```python
from build123d import *

# Parameters (mm, degrees)
SKETCH1_R                                           = 28
BOSS_EXTRUDE1_DEPTH                                 = 22
SKETCH2_R                                           = 10
BOSS_EXTRUDE2_DEPTH                                 = 22
SKETCH3_R                                           = 20
CUT_EXTRUDE1_DEPTH                                  = 16
CHAMFER1_SIZE                                       = 4
SKETCH4_R                                           = 4
CUT_EXTRUDE2_DEPTH                                  = 20
CBORE_FOR_M3_HEX_SOCKET_HEAD_CAP_SCREW1_D           = 3.4
CBORE_FOR_M3_HEX_SOCKET_HEAD_CAP_SCREW1_CBORE_D     = 6.5
CBORE_FOR_M3_HEX_SOCKET_HEAD_CAP_SCREW1_CBORE_DEPTH = 3.4
SKETCH7_R                                           = 26.5
SKETCH7_R_2                                         = 24.5
CUT_EXTRUDE3_DEPTH                                  = 4
M2_TAPPED_HOLE1_AT_2_COUNT                          = 2
M2_TAPPED_HOLE1_AT_2_PITCH                          = 11.388037985
M2_TAPPED_HOLE1_AT_3_COUNT                          = 2
M2_TAPPED_HOLE1_AT_3_PITCH                          = 22
M2_TAPPED_HOLE1_AT_4_COUNT                          = 2
M2_TAPPED_HOLE1_AT_4_PITCH                          = 31.112698372
M2_TAPPED_HOLE1_AT_5_COUNT                          = 2
M2_TAPPED_HOLE1_AT_5_PITCH                          = 38.105117767
M2_TAPPED_HOLE1_AT_6_COUNT                          = 2
M2_TAPPED_HOLE1_AT_6_PITCH                          = 42.500736357
M2_TAPPED_HOLE1_AT_7_COUNT                          = 2
M2_TAPPED_HOLE1_AT_7_PITCH                          = 44
M2_TAPPED_HOLE1_AT_8_COUNT                          = 2
M2_TAPPED_HOLE1_AT_8_PITCH                          = 42.500736357
M2_TAPPED_HOLE1_AT_9_COUNT                          = 2
M2_TAPPED_HOLE1_AT_9_PITCH                          = 38.105117767
M2_TAPPED_HOLE1_AT_10_COUNT                         = 2
M2_TAPPED_HOLE1_AT_10_PITCH                         = 31.112698372
M2_TAPPED_HOLE1_AT_11_COUNT                         = 2
M2_TAPPED_HOLE1_AT_11_PITCH                         = 22
M2_TAPPED_HOLE1_AT_12_COUNT                         = 2
M2_TAPPED_HOLE1_AT_12_PITCH                         = 11.388037985
SKETCH10_R                                          = 28
SKETCH10_R_2                                        = 24
CUT_EXTRUDE5_DEPTH                                  = 6
CUT_EXTRUDE5_DEPTH_BACK                             = 6
CHAMFER2_SIZE                                       = 1
M4_TAPPED_HOLE1_REACH                               = 60.172
M4_TAPPED_HOLE1_BORE_R                              = 1.65
CIRPATTERN1_COUNT                                   = 2
CIRPATTERN1_ANGLE                                   = 90


with BuildPart() as part:
    # Sketch1 → Boss-Extrude1 (new body)
    with BuildSketch(Plane.XY):
        Circle(SKETCH1_R)
    extrude(amount=BOSS_EXTRUDE1_DEPTH)

    # Sketch2 → Boss-Extrude2 (add)
    with BuildSketch(Plane.XY.offset(22)):
        Circle(SKETCH2_R)
    extrude(amount=BOSS_EXTRUDE2_DEPTH)

    # Sketch3 → Cut-Extrude1 (cut)
    with BuildSketch(Plane(origin=(0, 0, 0), x_dir=(-1, 0, 0), z_dir=(0, 0, -1))):
        Circle(SKETCH3_R)
    extrude(amount=-CUT_EXTRUDE1_DEPTH, mode=Mode.SUBTRACT)

    # Chamfer1
    chamfer1_edges = [part.edges().sort_by_distance(p)[0] for p in [
        (20, 0, 16),
    ]]
    chamfer(chamfer1_edges, length=CHAMFER1_SIZE)

    # Sketch4 → Cut-Extrude2 (cut)
    with BuildSketch(Plane.XY.offset(44)):
        Circle(SKETCH4_R)
    extrude(amount=-CUT_EXTRUDE2_DEPTH, mode=Mode.SUBTRACT)

    # CBORE for M3 Hex Socket Head Cap Screw1 (through all)
    with Locations(Plane(origin=(0, 0, 16), x_dir=(-1, 0, 0), z_dir=(0, 0, -1))):
        with Locations((0, 0)):
            CounterBoreHole(CBORE_FOR_M3_HEX_SOCKET_HEAD_CAP_SCREW1_D / 2, CBORE_FOR_M3_HEX_SOCKET_HEAD_CAP_SCREW1_CBORE_D / 2, CBORE_FOR_M3_HEX_SOCKET_HEAD_CAP_SCREW1_CBORE_DEPTH)

    # Sketch7 → Cut-Extrude3 (cut)
    with BuildSketch(Plane(origin=(0, 0, 0), x_dir=(-1, 0, 0), z_dir=(0, 0, -1))):
        Circle(SKETCH7_R)
        Circle(SKETCH7_R_2, mode=Mode.SUBTRACT)
    cut_extrude3 = extrude(amount=-CUT_EXTRUDE3_DEPTH, mode=Mode.SUBTRACT)

    # Mirror1: Cut-Extrude3 across plane
    add(cut_extrude3.mirror(Plane(origin=(0, 0, 11), x_dir=(1, 0, 0), z_dir=(0, 0, -1))), mode=Mode.SUBTRACT)

    # Sketch9 → M2 Tapped Hole1 (revolve, cut)
    with BuildSketch(Plane(origin=(0, 22, 0), x_dir=(0, 1, 0), z_dir=(1, 0, 0))):
        Polygon((0, 0), (0, 8.480688495), (0.8, 8), (0.8, 0), align=None)
    m2_tapped_hole1 = revolve(axis=Axis((0, 22, -6.35), (0, 0, 1)), mode=Mode.SUBTRACT)

    # M2 Tapped Hole1 at 2: M2 Tapped Hole1 ×2
    with Locations(*[Vector(-0.9659258262891051, -0.2588190451023836, 0) * (i * M2_TAPPED_HOLE1_AT_2_PITCH) for i in range(1, M2_TAPPED_HOLE1_AT_2_COUNT)]):
        add(m2_tapped_hole1, mode=Mode.SUBTRACT)

    # M2 Tapped Hole1 at 3: M2 Tapped Hole1 ×2
    with Locations(*[Vector(-0.8660254037845097, -0.4999999999998771, 0) * (i * M2_TAPPED_HOLE1_AT_3_PITCH) for i in range(1, M2_TAPPED_HOLE1_AT_3_COUNT)]):
        add(m2_tapped_hole1, mode=Mode.SUBTRACT)

    # M2 Tapped Hole1 at 4: M2 Tapped Hole1 ×2
    with Locations(*[Vector(-0.7071067811866479, -0.7071067811864472, 0) * (i * M2_TAPPED_HOLE1_AT_4_PITCH) for i in range(1, M2_TAPPED_HOLE1_AT_4_COUNT)]):
        add(m2_tapped_hole1, mode=Mode.SUBTRACT)

    # M2 Tapped Hole1 at 5: M2 Tapped Hole1 ×2
    with Locations(*[Vector(-0.500000000000123, -0.8660254037843677, 0) * (i * M2_TAPPED_HOLE1_AT_5_PITCH) for i in range(1, M2_TAPPED_HOLE1_AT_5_COUNT)]):
        add(m2_tapped_hole1, mode=Mode.SUBTRACT)

    # M2 Tapped Hole1 at 6: M2 Tapped Hole1 ×2
    with Locations(*[Vector(-0.2588190451026581, -0.9659258262890316, 0) * (i * M2_TAPPED_HOLE1_AT_6_PITCH) for i in range(1, M2_TAPPED_HOLE1_AT_6_COUNT)]):
        add(m2_tapped_hole1, mode=Mode.SUBTRACT)

    # M2 Tapped Hole1 at 7: M2 Tapped Hole1 ×2
    with Locations(*[(0, -i * M2_TAPPED_HOLE1_AT_7_PITCH, 0) for i in range(1, M2_TAPPED_HOLE1_AT_7_COUNT)]):
        add(m2_tapped_hole1, mode=Mode.SUBTRACT)

    # M2 Tapped Hole1 at 8: M2 Tapped Hole1 ×2
    with Locations(*[Vector(0.25881904510238346, -0.9659258262891051, 0) * (i * M2_TAPPED_HOLE1_AT_8_PITCH) for i in range(1, M2_TAPPED_HOLE1_AT_8_COUNT)]):
        add(m2_tapped_hole1, mode=Mode.SUBTRACT)

    # M2 Tapped Hole1 at 9: M2 Tapped Hole1 ×2
    with Locations(*[Vector(0.4999999999998768, -0.8660254037845098, 0) * (i * M2_TAPPED_HOLE1_AT_9_PITCH) for i in range(1, M2_TAPPED_HOLE1_AT_9_COUNT)]):
        add(m2_tapped_hole1, mode=Mode.SUBTRACT)

    # M2 Tapped Hole1 at 10: M2 Tapped Hole1 ×2
    with Locations(*[Vector(0.7071067811864471, -0.7071067811866479, 0) * (i * M2_TAPPED_HOLE1_AT_10_PITCH) for i in range(1, M2_TAPPED_HOLE1_AT_10_COUNT)]):
        add(m2_tapped_hole1, mode=Mode.SUBTRACT)

    # M2 Tapped Hole1 at 11: M2 Tapped Hole1 ×2
    with Locations(*[Vector(0.8660254037843675, -0.5000000000001233, 0) * (i * M2_TAPPED_HOLE1_AT_11_PITCH) for i in range(1, M2_TAPPED_HOLE1_AT_11_COUNT)]):
        add(m2_tapped_hole1, mode=Mode.SUBTRACT)

    # M2 Tapped Hole1 at 12: M2 Tapped Hole1 ×2
    with Locations(*[Vector(0.9659258262890317, -0.2588190451026578, 0) * (i * M2_TAPPED_HOLE1_AT_12_PITCH) for i in range(1, M2_TAPPED_HOLE1_AT_12_COUNT)]):
        add(m2_tapped_hole1, mode=Mode.SUBTRACT)

    # Sketch10 → Cut-Extrude5 (cut, two sides)
    with BuildSketch(Plane(origin=(0, 0, 11), x_dir=(-1, 0, 0), z_dir=(0, 0, -1))) as cut_extrude5_sk:
        Circle(SKETCH10_R)
        Circle(SKETCH10_R_2, mode=Mode.SUBTRACT)
    extrude(amount=CUT_EXTRUDE5_DEPTH, mode=Mode.SUBTRACT)
    extrude(cut_extrude5_sk.sketch, amount=-CUT_EXTRUDE5_DEPTH_BACK, mode=Mode.SUBTRACT)

    # Mirror2: M2 Tapped Hole1 across plane
    add(m2_tapped_hole1.mirror(Plane(origin=(0, 0, 11), x_dir=(1, 0, 0), z_dir=(0, 0, -1))), mode=Mode.SUBTRACT)

    # Mirror2 copy 1 sketch → Mirror2 copy 1 (revolve, cut)
    with BuildSketch(Plane(origin=(-11, 19.052558883, 22), x_dir=(0, 1, 0), z_dir=(1, 0, 0))):
        Polygon((0, 0), (0, -8.480688495), (0.8, -8), (0.8, 0), align=None)
    revolve(axis=Axis((-11, 19.052558883, 28.35), (0, 0, 1)), mode=Mode.SUBTRACT)

    # Mirror2 copy 2 sketch → Mirror2 copy 2 (revolve, cut)
    with BuildSketch(Plane(origin=(-19.052558883, 11, 22), x_dir=(0, 1, 0), z_dir=(1, 0, 0))):
        Polygon((0, 0), (0, -8.480688495), (0.8, -8), (0.8, 0), align=None)
    revolve(axis=Axis((-19.052558883, 11, 28.35), (0, 0, 1)), mode=Mode.SUBTRACT)

    # Mirror2 copy 3 sketch → Mirror2 copy 3 (revolve, cut)
    with BuildSketch(Plane(origin=(-22, 0, 22), x_dir=(0, 1, 0), z_dir=(1, 0, 0))):
        Polygon((0, 0), (0, -8.480688495), (0.8, -8), (0.8, 0), align=None)
    revolve(axis=Axis((-22, 0, 28.35), (0, 0, 1)), mode=Mode.SUBTRACT)

    # Mirror2 copy 4 sketch → Mirror2 copy 4 (revolve, cut)
    with BuildSketch(Plane(origin=(-19.052558883, -11, 22), x_dir=(0, 1, 0), z_dir=(1, 0, 0))):
        Polygon((0, 0), (0, -8.480688495), (0.8, -8), (0.8, 0), align=None)
    revolve(axis=Axis((-19.052558883, -11, 28.35), (0, 0, 1)), mode=Mode.SUBTRACT)

    # Mirror2 copy 5 sketch → Mirror2 copy 5 (revolve, cut)
    with BuildSketch(Plane(origin=(-11, -19.052558883, 22), x_dir=(0, 1, 0), z_dir=(1, 0, 0))):
        Polygon((0, 0), (0, -8.480688495), (0.8, -8), (0.8, 0), align=None)
    revolve(axis=Axis((-11, -19.052558883, 28.35), (0, 0, 1)), mode=Mode.SUBTRACT)

    # Mirror2 copy 6 sketch → Mirror2 copy 6 (revolve, cut)
    with BuildSketch(Plane(origin=(0, -22, 22), x_dir=(0, 1, 0), z_dir=(1, 0, 0))):
        Polygon((0, 0), (0, -8.480688495), (0.8, -8), (0.8, 0), align=None)
    revolve(axis=Axis((0, -22, 28.35), (0, 0, 1)), mode=Mode.SUBTRACT)

    # Mirror2 copy 7 sketch → Mirror2 copy 7 (revolve, cut)
    with BuildSketch(Plane(origin=(11, -19.052558883, 22), x_dir=(0, 1, 0), z_dir=(1, 0, 0))):
        Polygon((0, 0), (0, -8.480688495), (0.8, -8), (0.8, 0), align=None)
    revolve(axis=Axis((11, -19.052558883, 28.35), (0, 0, 1)), mode=Mode.SUBTRACT)

    # Mirror2 copy 8 sketch → Mirror2 copy 8 (revolve, cut)
    with BuildSketch(Plane(origin=(19.052558883, -11, 22), x_dir=(0, 1, 0), z_dir=(1, 0, 0))):
        Polygon((0, 0), (0, -8.480688495), (0.8, -8), (0.8, 0), align=None)
    revolve(axis=Axis((19.052558883, -11, 28.35), (0, 0, 1)), mode=Mode.SUBTRACT)

    # Mirror2 copy 9 sketch → Mirror2 copy 9 (revolve, cut)
    with BuildSketch(Plane(origin=(22, 0, 22), x_dir=(0, 1, 0), z_dir=(1, 0, 0))):
        Polygon((0, 0), (0, -8.480688495), (0.8, -8), (0.8, 0), align=None)
    revolve(axis=Axis((22, 0, 28.35), (0, 0, 1)), mode=Mode.SUBTRACT)

    # Mirror2 copy 10 sketch → Mirror2 copy 10 (revolve, cut)
    with BuildSketch(Plane(origin=(19.052558883, 11, 22), x_dir=(0, 1, 0), z_dir=(1, 0, 0))):
        Polygon((0, 0), (0, -8.480688495), (0.8, -8), (0.8, 0), align=None)
    revolve(axis=Axis((19.052558883, 11, 28.35), (0, 0, 1)), mode=Mode.SUBTRACT)

    # Mirror2 copy 11 sketch → Mirror2 copy 11 (revolve, cut)
    with BuildSketch(Plane(origin=(11, 19.052558883, 22), x_dir=(0, 1, 0), z_dir=(1, 0, 0))):
        Polygon((0, 0), (0, -8.480688495), (0.8, -8), (0.8, 0), align=None)
    revolve(axis=Axis((11, 19.052558883, 28.35), (0, 0, 1)), mode=Mode.SUBTRACT)

    # Chamfer2
    chamfer2_edges = [part.edges().sort_by_distance(p)[0] for p in [
        (-4, 0, 44),
        (-10, 0, 22),
        (-10, 0, 44),
    ]]
    chamfer(chamfer2_edges, length=CHAMFER2_SIZE)

    # M4 Tapped Hole1 bore (on position points) → M4 Tapped Hole1 (cut, up to next)
    with BuildSketch(Plane(origin=(0, 10, 34), x_dir=(1, 0, 0), z_dir=(0, 1, 0)), mode=Mode.PRIVATE) as m4_tapped_hole1_sk1:
        Circle(M4_TAPPED_HOLE1_BORE_R)
    m4_tapped_hole1_tool1 = extrude(m4_tapped_hole1_sk1.sketch, amount=-M4_TAPPED_HOLE1_REACH, mode=Mode.PRIVATE) & part.part
    m4_tapped_hole1 = m4_tapped_hole1_tool1.solids().sort_by_distance((0, 10, 34))[0]
    add(m4_tapped_hole1, mode=Mode.SUBTRACT)

    # CirPattern1: M4 Tapped Hole1 ×2 about axis
    cirpattern1_axis = Axis((0, 0, 24), (0, 0, -1))
    for i in range(1, CIRPATTERN1_COUNT):
        add(m4_tapped_hole1.rotate(cirpattern1_axis, i * CIRPATTERN1_ANGLE / (CIRPATTERN1_COUNT - 1)), mode=Mode.SUBTRACT)


solid = part.part
```
The model under review builds one solid part; all positions refer to its coordinate system, in mm. A direction names the side the tool comes from. Round coordinates to 2 decimals unless told otherwise and drop trailing zeros. Loops run counter-clockwise (first coordinate to the right, second up) from the corner with the lowest first, then second, coordinate; pieces in that order, holes last. Notation, with made-up numbers: (26, 64.25) -> (57, 64.25) arc R32 ccw to (57, 100.25) -> close; hole circle Ø4 at (-6.75, 88). An arc over 180 degrees is marked (long way). Answer as a JSON object with one key per item and string values. Group by question number.
1) For line 1 (Y direction, x = 0, z = 19.9); line 2 (Y direction, x = 0, z = 17.2); line 3 (Y direction, x = 0, z = 7.5), list the stretches that pass through material, from the lowest coordinate up. Write a range as [from, to].
2) We need section A-A on z = 34. Write out the cut boundary in (x, y), then the cut area to 3 significant figures.
3) For pin 1 Ø1 at (x, y) = (22, 0) entering from -Z; pin 2 Ø1.8 at (x, y) = (11, 19.05) entering from +Z; pin 3 Ø12 at (x, z) = (-8, 7) entering from +Y, all flat-tipped, find the tip position at first contact; note any pin that passes through.
4) We need section B-B on z = 7. Give the number of separate pieces and of enclosed holes in the cut face, then the cut area to 3 significant figures.
5) For faces 1 (the face through (10.965, 18.253, 3.944)), 2 (the face through (6.87, -0.89, 32.61)), 3 (the face through (-7.73, -23.43, 18)), list the 3-axis set-ups (+Z, -Z, +X, -X, +Y, -Y) from which the entire face can be reached by the end or side of a thin tool; tool diameter is ignored.
6) Mouldability with a two-part tool opening along Y and no side actions: class faces 4 (the face through (-3.2, -2.4, 33.6)), 5 (the face through (11, -5, 22)), 6 (the face through (-11.042, 19.185, 8.397)) as released by +Y, released by -Y, zero draft, split by the parting line, or undercut.
Result set:
{
 "1": {"line 1": "[-28, -26.5], [-24.5, -22.8], [-21.2, -1.7], [1.7, 21.2], [22.8, 24.5], [26.5, 28]", "line 2": "[-28, -22.8], [-21.2, -3.25], [3.25, 21.2], [22.8, 28]", "line 3": "[-24, -22.8], [-21.2, -20], [20, 21.2], [22.8, 24]"},
 "2": {"outline": "(-1.65, 3.64) -> (-1.65, 9.86) arc R10 ccw (long way) to (9.86, -1.65) -> (3.64, -1.65) arc R4 cw (long way) to start; (1.65, 3.64) arc R4 cw to (3.64, 1.65) -> (9.86, 1.65) arc R10 ccw to (1.65, 9.86) -> close", "area": "224 mm²"},
 "3": {"pin 1": "z = 8.18", "pin 2": "z = 22", "pin 3": "y = 27.9"},
 "4": {"separate pieces": "1", "enclosed holes": "13", "area": "529 mm²"},
 "5": {"face 1": "-Z", "face 2": "+X", "face 3": "+Z"},
 "6": {"face 4": "undercut", "face 5": "zero draft", "face 6": "undercut"}
}
